Read the model definition and answer for the solid it produces. Units are mm, in the model's axes. Face numbers are marked on the shaded views. A direction names the side the tool comes from. Coordinates: 2 decimals unless noted, no trailing zeros. Write each loop counter-clockwise with the first axis right and the second up, starting at its lowest first coordinate (ties: lowest second). Pieces come first, ordered by that corner, then holes. Notation, with made-up numbers: (68.25, 85) -> (84.25, 85) arc R28 ccw to (84.25, 122) -> close; hole circle Ø10 at (-39.5, 65.5). An arc over 180 degrees is marked (long way). Return JSON: item names as keys, results as strings.
from build123d import *

# Parameters (mm, degrees)
SKETCH_1_W          = 50
SKETCH_1_H          = 40
EXTRUDE_1_DEPTH     = 19
SKETCH_2_W          = 46
SKETCH_2_H          = 15
CUT_EXTRUDE_1_DEPTH = 38
SKETCH_3_W          = 40
SKETCH_3_H          = 2
CUT_EXTRUDE_2_DEPTH = 30
FILLET_1_R          = 6


with BuildPart() as part:
    # 스케치1 → 보스-돌출1 (new body)
    with BuildSketch(Plane.XY):
        Rectangle(SKETCH_1_W, SKETCH_1_H)
    extrude(amount=EXTRUDE_1_DEPTH)

    # 스케치2 → 컷-돌출1 (cut)
    with BuildSketch(Plane(origin=(0, 20, 0), x_dir=(1, 0, 0), z_dir=(0, 1, 0))):
        with Locations((0, -9.5)):
            Rectangle(SKETCH_2_W, SKETCH_2_H)
    extrude(amount=-CUT_EXTRUDE_1_DEPTH, mode=Mode.SUBTRACT)

    # 스케치3 → 컷-돌출2 (cut)
    with BuildSketch(Plane(origin=(0, 20, 0), x_dir=(1, 0, 0), z_dir=(0, 1, 0))):
        with Locations((0, -18)):
            Rectangle(SKETCH_3_W, SKETCH_3_H)
    extrude(amount=-CUT_EXTRUDE_2_DEPTH, mode=Mode.SUBTRACT)

    # 필렛1
    fillet_1_edges = [part.edges().sort_by_distance(p)[0] for p in [
        (23, -18, 9.5),
        (-23, -18, 9.5),
        (20, -10, 18),
        (-20, -10, 18),
        (25, -20, 9.5),
        (-25, -20, 9.5),
    ]]
    fillet(fillet_1_edges, radius=FILLET_1_R)


solid = part.part
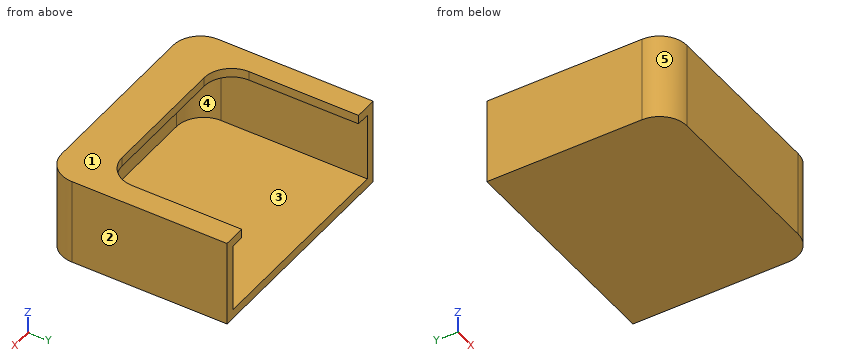
1. The part is cut by section C-C (z = 9.5). Determine the outline of the cut face in (x, y), then the cut area to 3 significant figures.
Taken from the geometry:
{"outline": "(-25, -14) arc R6 ccw to (-19, -20) -> (19, -20) arc R6 ccw to (25, -14) -> (25, 20) -> (23, 20) -> (23, -12) arc R6 cw to (17, -18) -> (-17, -18) arc R6 cw to (-23, -12) -> (-23, 20) -> (-25, 20) -> close", "area": "252 mm2"}
2. Flat-ended cylindrical pins translate along their axes: pin 1 Ø1 at (x, z) = (6, 17.5) entering from +Y; pin 2 Ø2 at (x, y) = (6.5, 12) entering from +Z; pin 3 Ø4.5 at (x, z) = (8.5, 9) entering from +Y. Find the tip coordinate at first contact, or state that the pin passes through.
Taken from the geometry:
{"pin 1": "stops at y = -10", "pin 2": "stops at z = 2", "pin 3": "stops at y = -18"}
3. For a pull along Z with two mould halves and no side action, classify the marked faces 1, 2 and 3 as +Z half, -Z half, draft (parallel to the pull), parting line (faces both ways), or undercut.
Taken from the geometry:
{"face 1": "+Z half", "face 2": "draft", "face 3": "undercut"}
4. The part is cut by section B-B (y = 14.5). Determine the outline of the cut face in (x, z), then the cut area to 3 significant figures.
Taken from the geometry:
{"outline": "(-25, 0) -> (25, 0) -> (25, 19) -> (20, 19) -> (20, 17) -> (23, 17) -> (23, 2) -> (-23, 2) -> (-23, 17) -> (-20, 17) -> (-20, 19) -> (-25, 19) -> close", "area": "180 mm2"}
5. A tool of negligible diameter and unlimited length cuts with its end or side. For the marked faces 4 and 5, from which of +Z, -Z, +X, -X, +Y, -Y can it reach the whole face along a straight path? Write none if from no direction.
Taken from the geometry:
{"face 4": "+Y", "face 5": "+Z, -Z, -X, -Y"}
6. Consider L1, parallel to X at y = -2.5, z = 7.75; L2, parallel to Z at x = 17.5, y = -12; L3, parallel to Y at x = 0, z = 5.5. Determine where each line is inside the solid, lowest interval first.
Taken from the geometry:
{"L1": "x = -25 to -23, 23 to 25", "L2": "z = 0 to 2, 17 to 19", "L3": "y = -20 to -18"}
7. The part is cut by section A-A (x = 3.5). Determine the outline of the cut face in (y, z).
Taken from the geometry:
{"outline": "(-20, 0) -> (20, 0) -> (20, 2) -> (-18, 2) -> (-18, 17) -> (-10, 17) -> (-10, 19) -> (-20, 19) -> close"}
